```python
from build123d import *

# Parameters (mm, degrees)
SKETCH_1_R               = 7.5
SKETCH_1_R_2             = 3
EXTRUDE_1_DEPTH          = 5
SKETCH_2_W               = 0.65965233
SKETCH_2_H               = 3
CUT_EXTRUDE_1_DEPTH      = 10
PATTERN_CIRCULAR_1_COUNT = 8


with BuildPart() as part:
    # Эскиз1 → Бобышка-Вытянуть1 (new body)
    with BuildSketch(Plane(origin=(0, 0, 0), x_dir=(1, 0, 0), z_dir=(0, 1, 0))):
        Circle(SKETCH_1_R)
        Circle(SKETCH_1_R_2, mode=Mode.SUBTRACT)
    extrude(amount=EXTRUDE_1_DEPTH)

    # Эскиз2 → Вырез-Вытянуть1 (cut)
    with BuildSketch(Plane(origin=(0, 5, 0), x_dir=(1, 0, 0), z_dir=(0, 1, 0))):
        with Locations((0, 5)):
            Rectangle(SKETCH_2_W, SKETCH_2_H)
    cut_extrude_1 = extrude(amount=-CUT_EXTRUDE_1_DEPTH, mode=Mode.SUBTRACT)

    # Круговой массив1: Вырез-Вытянуть1 ×8 about axis
    pattern_circular_1_axis = Axis((0, 0, 0), (0, 1, 0))
    for i in range(1, PATTERN_CIRCULAR_1_COUNT):
        add(cut_extrude_1.rotate(pattern_circular_1_axis, i * 360 / PATTERN_CIRCULAR_1_COUNT), mode=Mode.SUBTRACT)


solid = part.part
```
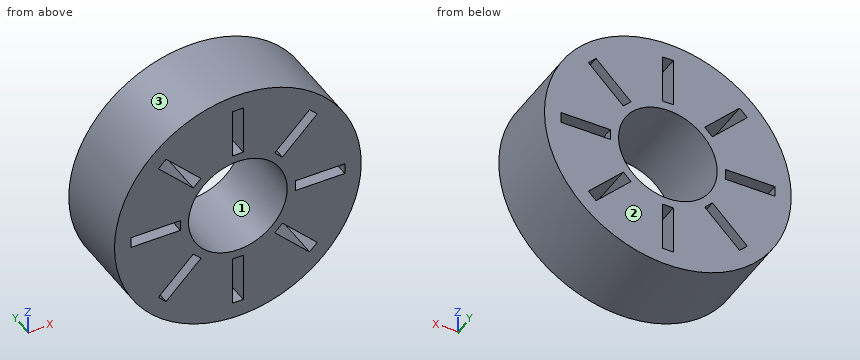
Verification items for the finished model (mm, model axes). Face numbers are marked on the shaded views. Round coordinates to 2 decimals unless told otherwise and drop trailing zeros. Write each loop counter-clockwise with the first axis right and the second up, starting at its lowest first coordinate (ties: lowest second). Pieces come first, ordered by that corner, then holes.
1. Draft check along X on the marked faces 1, 2 and 3. Enter one of: +X half, -X half, draft (parallel to the pull), parting line (faces both ways), or undercut.
2. Scan lines: L1, parallel to Z at x = 0, y = 3.45; L2, parallel to Z at x = -2.75, y = 4.45. Record each from-to range of solid material in increasing order.
3. Section check D-D on x = 0. Enter the section's corners in (y, z).
4. Section check A-A on z = 0. Enter the section's corners in (x, y).
5. Section check B-B on x = 6. Enter the section's corners in (y, z), plus the area to 3 significant figures.
6. Gauge pin test, flat ends, axial feed: P1, Ø2.5, axis at x = 5.5, y = 2.5, coming from the -Z side; P2, Ø1.5, axis at y = 2, z = -3.5, coming from the -X side; P3, Ø1.5, axis at y = 3.5, z = -4.5, coming from the -X side; P4, Ø2, axis at x = -2.5, z = 0.5, coming from the +Y side. Record the tip position at first contact, or that the pin passes through.
7. Section check C-C on y = 0.5. State how many separate pieces and enclosed holes the cut face has, plus the area to 3 significant figures.
Answer:
1. face 1: undercut
1. face 2: draft
1. face 3: parting line
2. L1: z = -7.5 to -6.5, -3.5 to -3, 3 to 3.5, 6.5 to 7.5
2. L2: z = -6.98 to -3.22, -2.28 to -1.2, 1.2 to 2.28, 3.22 to 6.98
3. outline: (0, -7.5) - (5, -7.5) - (5, -6.5) - (0, -6.5) - close; (0, -3.5) - (5, -3.5) - (5, -3) - (0, -3) - close; (0, 3) - (5, 3) - (5, 3.5) - (0, 3.5) - close; (0, 6.5) - (5, 6.5) - (5, 7.5) - (0, 7.5) - close
4. outline: (-7.5, 0) - (-6.5, 0) - (-6.5, 5) - (-7.5, 5) - close; (-3.5, 0) - (-3, 0) - (-3, 5) - (-3.5, 5) - close; (3, 0) - (3.5, 0) - (3.5, 5) - (3, 5) - close; (6.5, 0) - (7.5, 0) - (7.5, 5) - (6.5, 5) - close
5. outline: (0, -4.5) - (5, -4.5) - (5, -0.33) - (0, -0.33) - close; (0, 0.33) - (5, 0.33) - (5, 4.5) - (0, 4.5) - close
5. area: 41.7 mm2
6. P1: stops at z = -6.18
6. P2: stops at x = -6.98
6. P3: stops at x = -6.5
6. P4: stops at y = 5
7. separate pieces: 1
7. enclosed holes: 9
7. area: 133 mm2
